Here's the drawing with two shaded views (mm, measured from the low corner). I have some questions. A direction names the side the tool comes from. Coordinates: 2 decimals unless noted, no trailing zeros. Write each loop counter-clockwise with the first axis right and the second up, starting at its lowest first coordinate (ties: lowest second). Pieces come first, ordered by that corner, then holes. Notation, with made-up numbers: M 86,24 L 102,24 A10 cw 102,35 Z; hole C 79,-25.75 d4. An arc over 180 degrees is marked long. Use one line per item in the form item = value. Start each with the question number.
1. I want a section at D-D, the plane y = 7.25. List the corners of the cut face in (x, z) for me, plus the area to 4 significant figures.
2. I want a section at B-B, the plane y = 3.25. List the corners of the cut face in (x, z) for me.
3. On a 3-axis mill with a long thin cutter (end or side, diameter ignored), from which of +Z, -Z, +X, -X, +Y, -Y can I reach the whole of each face in a straight line? I mean the marked faces 1 and 2. Say none if no direction works.
4. I want a section at A-A, the plane x = 5. List the corners of the cut face in (y, z) for me, plus the area to 3 significant figures.
5. I want a section at C-C, the plane z = 1.35. List the corners of the cut face in (x, y) for me.
6. I'm going to push flat-ended pins straight in: pin 1 Ø1 at (x, z) = (2, 1.5) entering from +Y; pin 2 Ø0.9 at (y, z) = (3.5, 3) entering from +X. Where does each tip first touch, or does it pass through?
7. Please list where these lines run through material, in increasing order: line 1 along Z through (x, y) = (1.75, 1.75); line 2 along X through (y, z) = (4.75, 3.75). Write a range as [from, to].
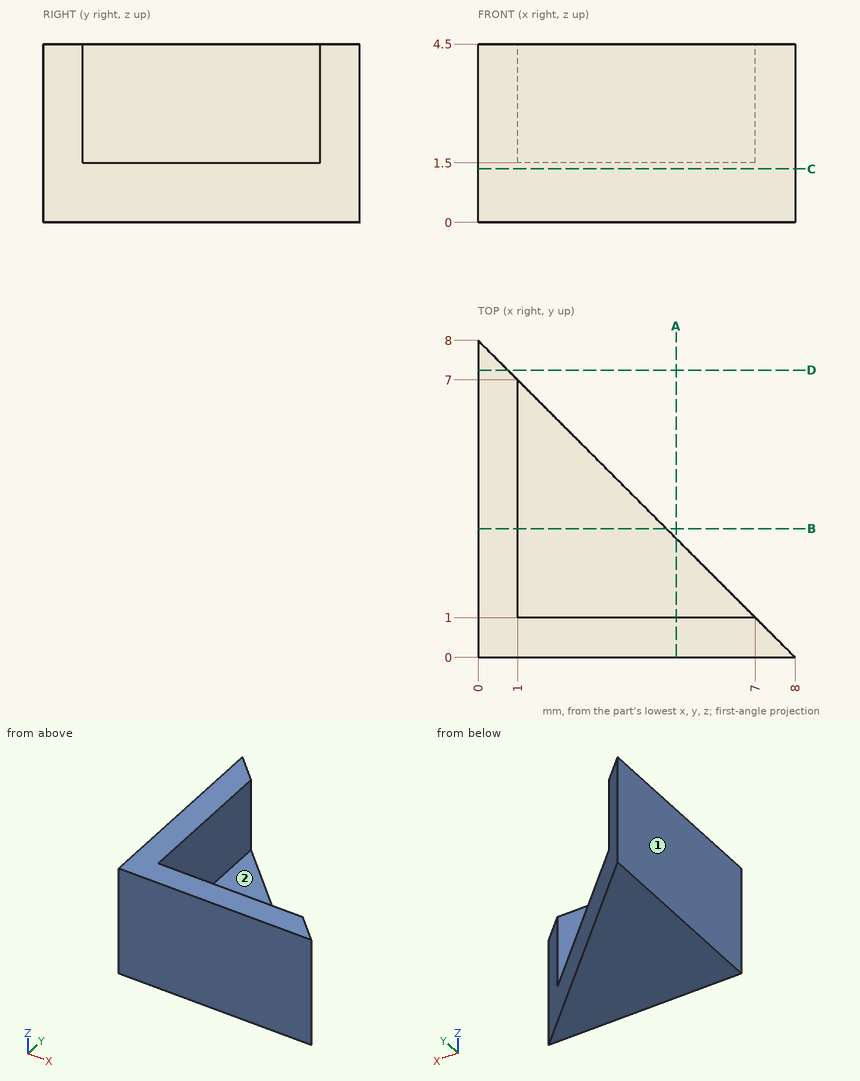
Answer list:
q1.outline = M 0,0 L 0.75,0 L 0.75,4.5 L 0,4.5 Z
q1.area = 3.375 mm²
q2.outline = M 0,0 L 4.75,0 L 4.75,1.5 L 1,1.5 L 1,4.5 L 0,4.5 Z
q3.face_1 = +Z, -Z, -X, +Y, -Y
q3.face_2 = +Z, +X, +Y
q4.outline = M 0,0 L 3,0 L 3,1.5 L 1,1.5 L 1,4.5 L 0,4.5 Z
q4.area = 7.50 mm²
q5.outline = M 0,0 L 8,0 L 0,8 Z
q6.pin_1 = 6.5
q6.pin_2 = 1
q7.line_1 = [0, 1.5]
q7.line_2 = [0, 1]
